The model under review builds one solid part; all positions refer to its coordinate system, in mm. Face numbers are marked on the shaded views. A direction names the side the tool comes from. Round coordinates to 2 decimals unless told otherwise and drop trailing zeros. Order: outer loops, then holes, each group sorted by start corner. A loop starts at its lowest first (then second) coordinate and runs counter-clockwise, first axis right, second up. Notation, with made-up numbers: M 32.5,43.25 L 60.5,43.25 A12 ccw 60.5,61.25 Z; hole C -4.75,-10 d2. An arc over 180 degrees is marked long. Use a Markdown table: item, result. Add a question column.
1. The part is to be moulded in two halves that separate along Z. For the marked faces 3, 4 and 5, say which applies: +Z half, -Z half, draft (parallel to the pull), parting line (faces both ways), or undercut.
2. Consider section C-C on z = 702. State the section outline as (x, y) points, then the cut area to 3 significant figures.
3. Insertion check: P1, Ø10, axis at y = -46, z = 604, coming from the +X side; P2, Ø10, axis at y = -6, z = 610, coming from the -X side; P3, Ø1, axis at x = 33, z = 430.5, coming from the -Y side. Each pin has a flat end and moves straight along its axis. Give the tip position at first contact, or say it passes through.
4. To check wall thickness, follow probe 1 along Y at (x, z) = (-21, 530); probe 2 along X at (y, z) = (46.5, 715.5); probe 3 along X at (y, z) = (-18, 564). State the ranges of each line that lie inside material, in increasing order.
5. Consider section B-B on x = 90.5. State the section outline as (y, z) points.
6. Consider section A-A on y = 47. State the section outline as (x, z) points (3 decimals), then the cut area to 3 significant figures.
7. For the marked faces 1 and 2, list the 3-axis set-ups (+Z, -Z, +X, -X, +Y, -Y) from which the entire face can be reached by the end or side of a thin tool; tool diameter is ignored.
from build123d import *

# Parameters (mm, degrees)
MAIN_EXTRUDE_DEPTH = 65.09
SHELL1_T           = -5


with BuildPart() as part:
    # Sketch1 → Main extrude (new, symmetric)
    with BuildSketch(Plane(origin=(0, 0, 0), x_dir=(1, 0, 0), z_dir=(0, 1, 0))):
        Polygon((0, 0), (-117.055, -880.2309966), (117.055, -880.2309966), align=None)
    extrude(amount=MAIN_EXTRUDE_DEPTH, both=True)

    # Shell1
    shell1_openings = [part.faces().sort_by_distance(p)[0] for p in [
        (0, -65.09, 586.8206644),
    ]]
    offset(amount=SHELL1_T, openings=shell1_openings, kind=Kind.INTERSECTION)


solid = part.part
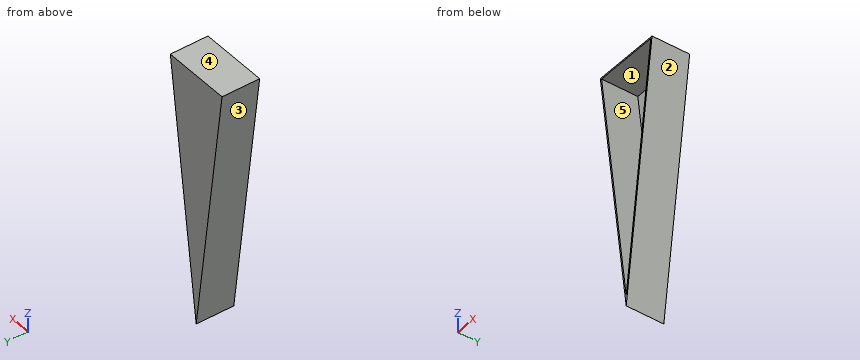
Answer block:
| question | item | result |
|---|---|---|
| 1 | face 3 | -Z half |
| 1 | face 4 | +Z half |
| 1 | face 5 | undercut |
| 2 | outline | M -93.35,-65.09 L -88.31,-65.09 L -88.31,60.09 L 88.31,60.09 L 88.31,-65.09 L 93.35,-65.09 L 93.35,65.09 L -93.35,65.09 Z |
| 2 | area | 2,200 mm^2 |
| 3 | P1 | x = 80.99 |
| 3 | P2 | x = -81.78 |
| 3 | P3 | y = 60.09 |
| 4 | probe 1 | 60.09 to 65.09 |
| 4 | probe 2 | -95.15 to -90.1, 90.1 to 95.15 |
| 4 | probe 3 | -75 to -69.96, 69.96 to 75 |
| 5 | outline | M -65.09,680.54 L 65.09,680.54 L 65.09,880.23 L -65.09,880.23 L -65.09,875.23 L 60.09,875.23 L 60.09,718.47 L -65.09,718.47 Z |
| 6 | outline | M -117.055,880.231 L 0,0 L 117.055,880.231 Z; hole M -111.346,875.231 L 0,37.93 L 111.346,875.231 Z |
| 6 | area | 9,810 mm^2 |
| 7 | face 1 | -Y |
| 7 | face 2 | -Z, +X, +Y, -Y |
